Autodesk Fusion 360 part; units mm, degrees
sketch "Sketch4" plane through (0, 0, 0) normal (1, 0, 0) x (0, 1, 0)
  line L0 (-93.8909, 93.8909) -> (-38.8909, 93.8909)
  line L1 (-38.8909, 93.8909) -> (0, 55)
  line L2 (0, 55) -> (0, 0)
  line L3 (0, 0) -> (-20, 0)
  line L4 (-93.8909, 93.8909) -> (-93.8909, 73.8909)
  line L5 (-93.8909, 73.8909) -> (-20, 0)
  line L6 (-16.4645, 23.5355) -> (-71.4645, 78.5355)
  arc A0 (-71.4645, 78.5355) -> (-78.5355, 71.4645) centre (-75, 75) ccw
  line L7 (-78.5355, 71.4645) -> (-23.5355, 16.4645)
  arc A1 (-23.5355, 16.4645) -> (-16.4645, 23.5355) centre (-20, 20) ccw
  line L8 (-20, 20) -> (-75, 75) construction
  circle A2 centre (-8, 10) radius 2
  circle A3 centre (-8, 45) radius 2
  line L9 (-8, 45) -> (-8, 10) construction
  line L10 (0, 27.5) -> (-8, 27.5) construction
  circle A4 centre (-8, 27.5) radius 2
  dimension "d15" = 55
  dimension "d16" = 135
  dimension "d17" = 55
  dimension "d18" = 55
  dimension "d19" = 20
  dimension "d20" = 20
  dimension "d21" = 10
  dimension "d22" = 4
  dimension "d23" = 4
  dimension "d24" = 8
  dimension "d25" = 35
  dimension "d35" = 4
extrude "Extrude1" add sketch "Sketch4" along normal blind 4
sketch "Sketch5" plane through (0, 0, 93.8909) normal (0, 0, 1) x (-1, 0, 0)
  line L0 (0, 38.8909) -> (0, 93.8909)
  line L1 (0, 93.8909) -> (-4, 93.8909)
  line L2 (-4, 93.8909) -> (-4, 38.8909)
  line L3 (-4, 38.8909) -> (0, 38.8909)
  line L4 (0, 93.8909) -> (-19, 93.8909)
  line L5 (-19, 93.8909) -> (-19, 38.8909)
  line L6 (-19, 38.8909) -> (0, 38.8909)
  line L7 (0, 38.8909) -> (0, 93.8909)
  circle A0 centre (-9.5, 83.8909) radius 2
  circle A1 centre (-9.5, 48.8909) radius 2
  line L8 (-9.5, 83.8909) -> (-9.5, 48.8909) construction
  line L9 (-9.5, 66.3909) -> (0, 66.3909) construction
  line L10 (-9.5, 48.8909) -> (-9.5, 38.8909) construction
  dimension "d28" = 55
  dimension "d30" = 4
  dimension "d31" = 4
  dimension "d32" = 35
  dimension "d36" = 19
extrude "Extrude3" add sketch "Sketch5" against normal blind 4 contours L2 L4 L5 L6
For this review, take the finished solid that the model builds, in its own axes (mm). A direction names the side the tool comes from. Give positions to 0.01 mm unless a question says otherwise; leave off trailing zeros. Write each loop counter-clockwise with the first axis right and the second up, starting at its lowest first coordinate (ties: lowest second). Pieces come first, ordered by that corner, then holes.
Item 1: Take a section at A-A (x = 9.5). Give the boundary of the cut face in (y, z), and give its area (3 significant figures).
Item 2: Wall thickness on probe 1 along Y at (x, z) = (9.5, 93.15); probe 2 along Z at (x, y) = (1.4, -8); probe 3 along Z at (x, y) = (14.5, -86): over which ranges is each line inside the solid? List them lowest first.
Item 3: Take a section at B-B (y = -33). Give the boundary of the cut face in (x, z), and give its area (3 significant figures).
Item 4: Insertion check: P1, Ø1, axis at x = 12, y = -61.5, coming from the -Z side; P2, Ø2, axis at y = -76, z = 62, coming from the +X side; P3, Ø3.5, axis at y = -8, z = 27.5, coming from the +X side; P4, Ø1.2, axis at x = 15, z = 93, coming from the +Y side. Each pin has a flat end and moves straight along its axis. Give the tip position at first contact, or say it passes through.
Item 5: The part is to be moulded in two halves that separate along Y. For faces 3 (the face through (12, -67, 89.891)), 4 (the face through (12, -38.891, 92)), 5 (the face through (1.97, -43.58, 50.65)), say which applies: +Y half, -Y half, draft (parallel to the pull), parting line (faces both ways), or undercut.
Item 6: Take a section at C-C (z = 39.5). Give the boundary of the cut face in (x, y).
Item 7: Machinability: for faces 1 (the face through (2, 0, 28)), 2 (the face through (1.97, -51.42, 44.35)), which of the approach directions +Z, -Z, +X, -X, +Y, -Y give a long, thin tool a straight path to every point of the face, cutting with its end or side? Answer none if there is none.
Item 8: Take a section at D-D (y = -57.5). Give the boundary of the cut face in (x, z), and give its area (3 significant figures).
Established:
1. outline: (-93.89, 89.89) - (-85.89, 89.89) - (-85.89, 93.89) - (-93.89, 93.89) - close; (-81.89, 89.89) - (-50.89, 89.89) - (-50.89, 93.89) - (-81.89, 93.89) - close; (-46.89, 89.89) - (-38.89, 89.89) - (-38.89, 93.89) - (-46.89, 93.89) - close
1. area: 188 mm2
2. probe 1: y = -93.89 to -85.89, -81.89 to -50.89, -46.89 to -38.89
2. probe 2: z = 0 to 8, 12 to 25.5, 29.5 to 43, 47 to 63
2. probe 3: z = 89.89 to 93.89
3. outline: (0, 13) - (4, 13) - (4, 25.93) - (0, 25.93) - close; (0, 40.07) - (4, 40.07) - (4, 88) - (0, 88) - close
3. area: 243 mm2
4. P1: stops at z = 89.89
4. P2: stops at x = 4
4. P3: passes through
4. P4: stops at y = -38.89
5. face 3: draft
5. face 4: +Y half
5. face 5: undercut
6. outline: (0, -59.5) - (4, -59.5) - (4, -46.57) - (0, -46.57) - close; (0, -32.43) - (4, -32.43) - (4, 0) - (0, 0) - close
7. face 1: +Z, -Z, +X, -X, +Y
7. face 2: +X, -X
8. outline: (0, 37.5) - (4, 37.5) - (4, 50.43) - (0, 50.43) - close; (0, 64.57) - (4, 64.57) - (4, 89.89) - (19, 89.89) - (19, 93.89) - (0, 93.89) - close
8. area: 229 mm2
